Source: CAD feature listing. Evaluate the final solid. Frame: model axes, mm. Face numbers are marked on the shaded views. A direction names the side the tool comes from. Give positions to 0.01 mm unless a question says otherwise; leave off trailing zeros. Loops run counter-clockwise (first coordinate to the right, second up) from the corner with the lowest first, then second, coordinate; pieces in that order, holes last. Notation, with made-up numbers: M 82,71.5 L 127,71.5 A8 ccw 127,78.5 Z; hole C -22,76 d11. An arc over 180 degrees is marked long. Answer in a Markdown table with one row per item.
```python
from build123d import *

# Parameters (mm, degrees)
F2_R = 25.7548302834
F4_R = 11.650994652


# Not quite as in the source:
# - a fillet or chamfer that OpenCascade refuses, or shapes differently, is made with other operations: its cross-section is extruded or revolved along the edge and cut away or added


with BuildPart() as f1:
    # F0 (on Front) → F1 (revolve)
    with BuildSketch(Plane.XZ):
        Polygon((0, 0), (0, 437.0113793103), (-61.3251142204, 437.0113793103), (-61.3251142204, 406.9045186043), (-39.9097763002, 406.9045186043), (-39.9097763002, 374.7815191746), (-68.7381178141, 374.7815191746), (-68.7381178141, 355.0135195255), (-48.9701107144, 355.0135195255), (-48.9701107144, 347.6004898548), (-76.974786818, 347.6004898548), (-76.974786818, 313.006490469), (-94.2717939615, 313.006490469), (-94.2717939615, 270.1758146286), (-107.95, 270.1758146286), (-107.95, 207.5771391392), (-83.5641175508, 193.5748010874), (-83.5641175508, 154.8624634743), (-68.7381178141, 154.8624634743), (-62.401818486, 36.0568519682), (-39.6875, 36.0568519682), (-39.6875, 0), align=None)
    revolve(axis=Axis((0, 0, 218.5056896552), (0, 0, -1)))

    # F2
    f2_edges = [f1.edges().sort_by_distance(p)[0] for p in [
        (76.974787, 0, 347.60049),
    ]]
    fillet(f2_edges, radius=F2_R)

    # F3: fillet of radius 19.0095175901 on 1 edges, made by hand

    # F3_s1 → F3_t2 (revolve, cut)
    with BuildSketch(Plane.XZ):
        with BuildLine():
            ThreePointArc((-76.974786818, 313.006490469), (-89.296444613, 306.8962751619), (-94.2717939615, 294.0742674886))
            Line((-94.2717939615, 294.0742674886), (-94.2717939615, 313.006490469))
            Line((-94.2717939615, 313.006490469), (-76.974786818, 313.006490469))
        make_face()
    revolve(axis=Axis((0, 0, 313.006490469), (0, 0, -1)), mode=Mode.SUBTRACT)

    # F4
    f4_edges = [f1.edges().sort_by_distance(p)[0] for p in [
        (107.95, 0, 270.175815),
    ]]
    fillet(f4_edges, radius=F4_R)


solid = f1.part
```
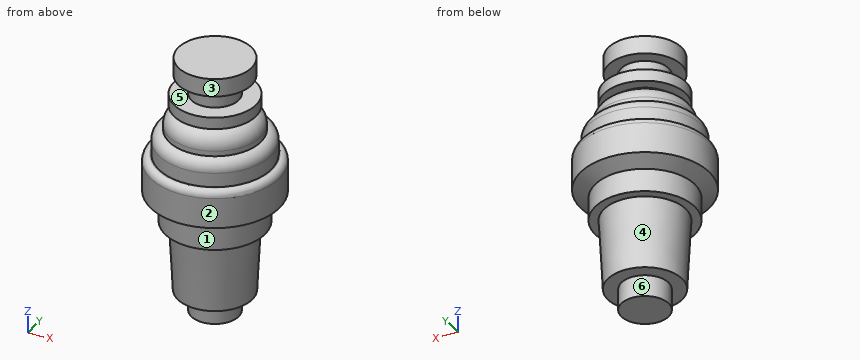
Q1. Mould query, pull axis Z, two halves, no side actions, for the marked faces 4, 5 and 6. Classes: +Z half, -Z half, draft (parallel to the pull), parting line (faces both ways), or undercut.
Values follow:
| item | result |
|---|---|
| face 4 | -Z half |
| face 5 | undercut |
| face 6 | draft |
Q2. Contact query for flat-ended pins moving along their axis: pin 1 Ø1 at (x, z) = (-44, 164.5) entering from -Y; pin 2 Ø4 at (x, z) = (54, 155.5) entering from -Y; pin 3 Ø1.5 at (x, z) = (3.5, 89.5) entering from -Y. Output: stop coordinate, or through.
Values follow:
| item | result |
|---|---|
| pin 1 | y = -71.35 |
| pin 2 | y = -65.41 |
| pin 3 | y = -65.21 |
Q3. Section query B-B (z = 123.5). Output: boundary loops of the cut face in (x, y).
Values follow:
| item | result |
|---|---|
| outline | C 0,0 d134.13 |
Q4. Ray query, probe 1 along Z at (x, y) = (2, -53); probe 2 along Z at (x, y) = (61, 11); probe 3 along Y at (x, z) = (10, 118). Return the intervals inside material, ascending. Write a range as from..to.
Values follow:
| item | result |
|---|---|
| probe 1 | 36.06..347.54, 355.01..374.78, 406.9..437.01 |
| probe 2 | 36.06..345.24, 355.01..374.78 |
| probe 3 | -66.02..66.02 |
Q5. Reachability of the marked faces 1, 2 and 3 from +Z, -Z, +X, -X, +Y, -Y: full face, straight path, thin tool, end or side. Return the list, or none.
Values follow:
| item | result |
|---|---|
| face 1 | -Z |
| face 2 | +Z, -Z |
| face 3 | +Z |
Q6. Section query A-A (z = 253.5). Output: boundary loops of the cut face in (x, y).
Values follow:
| item | result |
|---|---|
| outline | C 0,0 d215.9 |
